Autodesk Inventor part; units mm, degrees
ref_plane "YZ Plane" through (0, 0, 0) normal (1, 0, 0) x (0, 1, 0)
ref_plane "XZ Plane" through (0, 0, 0) normal (0, 1, 0) x (-1, 0, 0)
ref_plane "XY Plane" through (0, 0, 0) normal (0, 0, 1) x (1, 0, 0)
sketch "Sketch1" plane through (0, 0, 0) normal (0, 0, 1) x (1, 0, 0)
  circle A0 centre (13, 16) radius 1.425
  circle A1 centre (13, 6.05) radius 1.425
  circle A2 centre (40, 6.05) radius 1.425
  circle A3 centre (40, 16) radius 1.425
  line L0 (45, 1.05) -> (8, 1.05)
  line L1 (8, 1.05) -> (8, 21)
  line L2 (8, 21) -> (45, 21)
  line L3 (45, 21) -> (45, 1.05)
  point P0 (0, 0)
  dimension "d24" = 9.95
  dimension "d27" = 9.95
  dimension "d31" = 5
  dimension "d32" = 5
  dimension "d33" = 5
  dimension "d34" = 5
  dimension "d40" = 5
  dimension "d41" = 5
  dimension "d42" = 5
  dimension "d43" = 27
extrude "Extrusion1" add sketch "Sketch1" along normal blind 3.3
properties part number "Muñeca2"
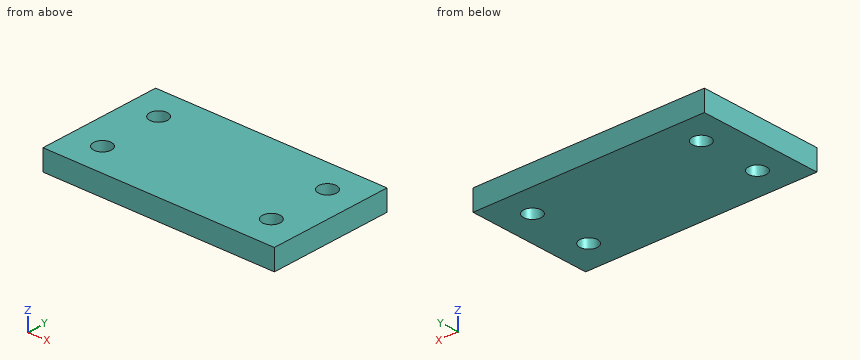
Geometry: final body of the model. Coordinates: model frame, mm. Round coordinates to 2 decimals unless told otherwise and drop trailing zeros. Write each loop counter-clockwise with the first axis right and the second up, starting at its lowest first coordinate (ties: lowest second). Pieces come first, ordered by that corner, then holes. Notation, with made-up numbers: (57.25, -8) -> (96.25, -8) arc R28 ccw to (96.25, 19) -> close; hole circle Ø10 at (18.25, 1.25). An arc over 180 degrees is marked (long way). Return JSON: item names as keys, results as strings.
Q1. Section C-C on y = 16. Return the cut outline in (x, z) (3 decimals).
From the geometry:
{"outline": "(8, 0) -> (11.575, 0) -> (11.575, 3.3) -> (8, 3.3) -> close; (14.425, 0) -> (38.575, 0) -> (38.575, 3.3) -> (14.425, 3.3) -> close; (41.425, 0) -> (45, 0) -> (45, 3.3) -> (41.425, 3.3) -> close"}
Q2. First-contact query: pin 1 Ø2.5 at (x, y) = (13, 16) entering from +Z. Flat tip, straight axial feed; report the tip coordinate or a pass-through.
From the geometry:
{"pin 1": "through"}
Q3. Section A-A on x = 40. Return the cut outline in (y, z) (3 decimals), and give its area (3 significant figures).
From the geometry:
{"outline": "(1.05, 0) -> (4.625, 0) -> (4.625, 3.3) -> (1.05, 3.3) -> close; (7.475, 0) -> (14.575, 0) -> (14.575, 3.3) -> (7.475, 3.3) -> close; (17.425, 0) -> (21, 0) -> (21, 3.3) -> (17.425, 3.3) -> close", "area": "47.0 mm2"}
Q4. Ray query, line 1 (Y direction, x = 40, z = 1.9) (3 decimals); line 2 (X direction, y = 6, z = 0.95); line 3 (X direction, y = 4.75, z = 0.65). Return the intervals inside material, ascending.
From the geometry:
{"line 1": "1.05 to 4.625, 7.475 to 14.575, 17.425 to 21", "line 2": "8 to 11.58, 14.42 to 38.58, 41.42 to 45", "line 3": "8 to 12.42, 13.58 to 39.42, 40.58 to 45"}
Q5. Section B-B on z = 1.5. Return the cut outline in (x, y) (3 decimals).
From the geometry:
{"outline": "(8, 1.05) -> (45, 1.05) -> (45, 21) -> (8, 21) -> close; hole circle Ø2.85 at (13, 6.05); hole circle Ø2.85 at (13, 16); hole circle Ø2.85 at (40, 6.05); hole circle Ø2.85 at (40, 16)"}
